```python
from build123d import *

# Parameters (mm, degrees)
F0_W     = 50
F0_H     = 50
F0_W_2   = 42.043511
F0_H_2   = 42.086583
F1_DEPTH = 750
F2_W     = 150
F2_H     = 150
F3_DEPTH = 5
F4_R     = 6.25
F5_DEPTH = 25


with BuildPart() as f1:
    # F0 (on Front) → F1 (new body)
    with BuildSketch(Plane.XZ):
        with Locations((-48.019424, 25)):
            Rectangle(F0_W, F0_H)
        with Locations((-48.149473, 25.268396)):
            Rectangle(F0_W_2, F0_H_2, mode=Mode.SUBTRACT)
    extrude(amount=F1_DEPTH)

    # F2 (on Front) → F3 (join)
    with BuildSketch(Plane.XZ):
        with Locations((-50.123258, 24.859246)):
            Rectangle(F2_W, F2_H)
    extrude(amount=F3_DEPTH)

    # F4 (on face) → F5 (cut)
    with BuildSketch(Plane(origin=(0, 0, 0), x_dir=(1, 0, 0), z_dir=(0, 0, -1))):
        with Locations((-50.928246, 550)):
            Circle(F4_R)
    extrude(amount=-F5_DEPTH, mode=Mode.SUBTRACT)


solid = f1.part
```
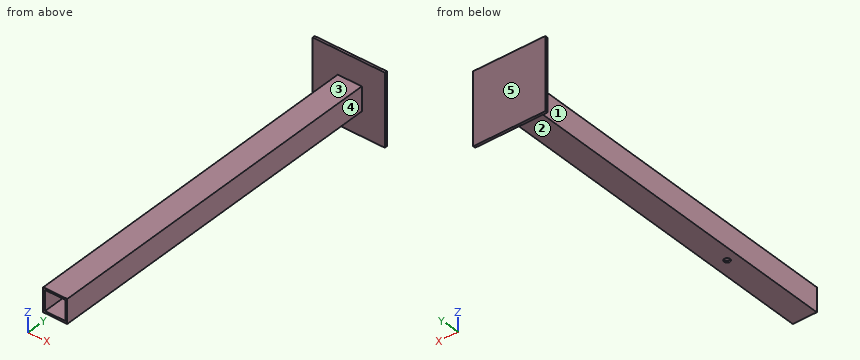
Model file for the job. Use its own axes, mm. Face numbers are marked on the shaded views. A direction names the side the tool comes from. Give positions to 0.01 mm unless a question says otherwise; leave off trailing zeros. Order: outer loops, then holes, each group sorted by start corner. A loop starts at its lowest first (then second) coordinate and runs counter-clockwise, first axis right, second up.
1) Pin check, flat tips, straight feed: pin 1 (25 mm diameter, centred on y = -462, z = 17, fed in from -X); pin 2 (3 mm diameter, centred on x = -66, y = -417.5, fed in from -Z); pin 3 (8 mm diameter, centred on x = -46.5, y = -308.5, fed in from +Z). Stop position of each tip, or through.
2) 3-axis set-ups, long thin cutter, end or side, ignore diameter. For the marked faces 4 and 5: which of +Z, -Z, +X, -X, +Y, -Y reach the whole face in a straight line?
3) Saw through at C-C, the plane z = -36.5. Write the cut outline in (x, y), then the cut area to 3 significant figures.
4) Saw through at B-B, the plane y = -550. Write the cut outline in (x, z), then the cut area to 3 significant figures.
5) Saw through at A-A, the plane y = -701. Write the cut outline in (x, z), then the cut area to 3 significant figures.
6) Saw through at D-D, the plane x = 10. Write the cut outline in (y, z), then the cut area to 3 significant figures.
7) Wall check: probe 1 along Z at (x, y) = (-31, -336.5); probe 2 along X at (y, z) = (-550, 3); probe 3 along X at (y, z) = (-519.5, 44). Give the ranges that are in metal, low to high.
8) Mould opens along Z. For the marked faces 1, 2 and 3 say: +Z half, -Z half, draft (parallel to the pull), parting line (faces both ways), or undercut.
Computed:
1. pin 1: stops at x = -73.02
1. pin 2: stops at z = 0
1. pin 3: stops at z = 50
2. face 4: +Z, -Z, +X, -Y
2. face 5: +Z, -Z, +X, -X, +Y
3. outline: (-125.12, -5) - (24.88, -5) - (24.88, 0) - (-125.12, 0) - close
3. area: 750 mm2
4. outline: (-73.02, 0) - (-57.18, 0) - (-57.18, 4.23) - (-69.17, 4.23) - (-69.17, 46.31) - (-27.13, 46.31) - (-27.13, 4.23) - (-44.68, 4.23) - (-44.68, 0) - (-23.02, 0) - (-23.02, 50) - (-73.02, 50) - close
4. area: 678 mm2
5. outline: (-73.02, 0) - (-23.02, 0) - (-23.02, 50) - (-73.02, 50) - close; hole (-69.17, 4.23) - (-27.13, 4.23) - (-27.13, 46.31) - (-69.17, 46.31) - close
5. area: 731 mm2
6. outline: (-5, -50.14) - (0, -50.14) - (0, 99.86) - (-5, 99.86) - close
6. area: 750 mm2
7. probe 1: z = 0 to 4.23, 46.31 to 50
7. probe 2: x = -73.02 to -57.18, -44.68 to -23.02
7. probe 3: x = -73.02 to -69.17, -27.13 to -23.02
8. face 1: draft
8. face 2: -Z half
8. face 3: +Z half
